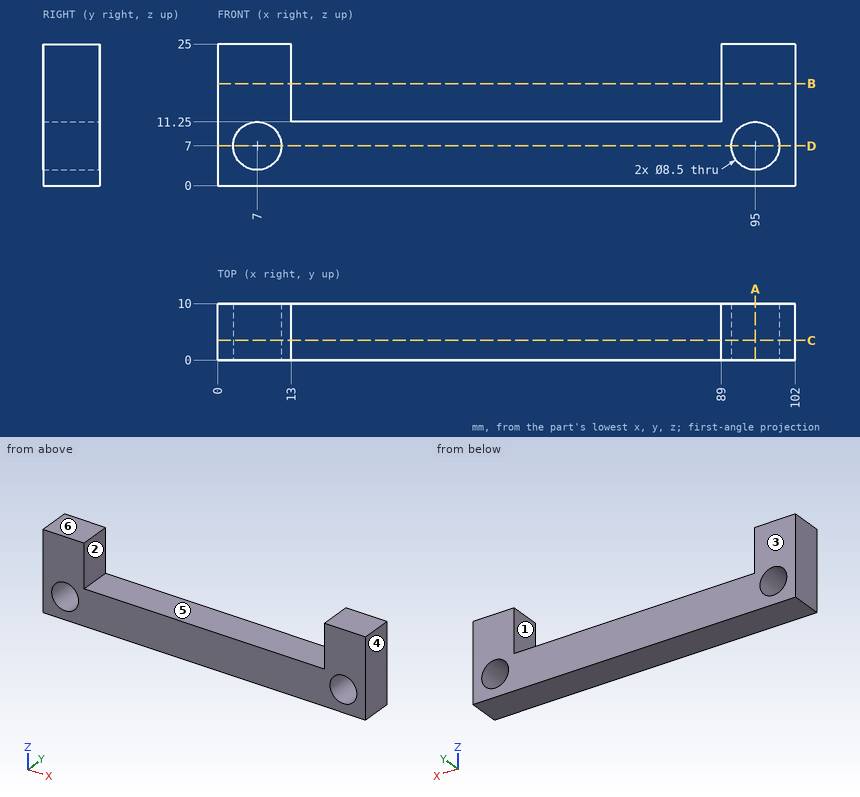
Check sheet for the drawn part. Datum: minimum x, y, z corner. Units: mm. A direction names the side the tool comes from. Give positions to 0.01 mm unless a question says otherwise; leave off trailing zeros. Order: outer loops, then holes, each group sorted by start corner. A loop starts at its lowest first (then second) coordinate and runs counter-clockwise, first axis right, second up. Notation, with made-up numbers: (86, -26.75) - (99, -26.75) arc R13 cw to (99, -15.75) - close; hole circle Ø4 at (51.5, -31). An arc over 180 degrees is marked (long way). Answer in a Markdown table with one row per item. Add a question column.
Q1. Mould release check, pull along X, two halves, no side actions. Record for the marked faces 1, 2, 3 and 4: pulls with the +X half, pulls with the -X half, needs draft (parallel to the pull), parting line crosses it, or undercut.
Q2. Cross-section at A-A, the plane x = 95. Enter the section's corners in (y, z), then the cut area to 3 significant figures.
Q3. Gauge pin test, flat end, axial feed: pin 1 (3 mm diameter, centred on x = 42, y = 6.5, fed in from +Z). Record the tip position at first contact, or that the pin passes through.
Q4. Cross-section at C-C, the plane y = 3.5. Enter the section's corners in (x, z), then the cut area to 3 significant figures.
Q5. Material ranges on probe 1 along X at (y, z) = (5, 7); probe 2 along X at (y, z) = (8, 20.25); probe 3 along Z at (x, y) = (95, 5.75), recorded low to high. Write a range as from..to.
Q6. Cross-section at B-B, the plane z = 18. Enter the section's corners in (x, y), then the cut area to 3 significant figures.
Q7. Tool access check on the marked faces 5 and 6. Record the directions out of +Z, -Z, +X, -X, +Y, -Y that give a thin tool (end or side, any length) a straight path to the whole face; none if there is none.
Q8. Cross-section at D-D, the plane z = 7. Enter the section's corners in (x, y).
Check values:
| question | item | result |
|---|---|---|
| 1 | face 1 | undercut |
| 1 | face 2 | undercut |
| 1 | face 3 | needs draft |
| 1 | face 4 | pulls with the +X half |
| 2 | outline | (0, 0) - (10, 0) - (10, 2.75) - (0, 2.75) - close; (0, 11.25) - (10, 11.25) - (10, 25) - (0, 25) - close |
| 2 | area | 165 mm^2 |
| 3 | pin 1 | stops at z = 11.25 |
| 4 | outline | (0, 0) - (102, 0) - (102, 25) - (89, 25) - (89, 11.25) - (13, 11.25) - (13, 25) - (0, 25) - close; hole circle Ø8.5 at (7, 7); hole circle Ø8.5 at (95, 7) |
| 4 | area | 1,390 mm^2 |
| 5 | probe 1 | x = 0..2.75, 11.25..90.75, 99.25..102 |
| 5 | probe 2 | x = 0..13, 89..102 |
| 5 | probe 3 | z = 0..2.75, 11.25..25 |
| 6 | outline | (0, 0) - (13, 0) - (13, 10) - (0, 10) - close; (89, 0) - (102, 0) - (102, 10) - (89, 10) - close |
| 6 | area | 260 mm^2 |
| 7 | face 5 | +Z, +Y, -Y |
| 7 | face 6 | +Z, +X, -X, +Y, -Y |
| 8 | outline | (0, 0) - (2.75, 0) - (2.75, 10) - (0, 10) - close; (11.25, 0) - (90.75, 0) - (90.75, 10) - (11.25, 10) - close; (99.25, 0) - (102, 0) - (102, 10) - (99.25, 10) - close |
